Job drawing, mm, ordinate dimensions from the low corner. One solid piece. A direction names the side the tool comes from. Give positions to 0.01 mm unless a question says otherwise; leave off trailing zeros. Write each loop counter-clockwise with the first axis right and the second up, starting at its lowest first coordinate (ties: lowest second). Pieces come first, ordered by that corner, then holes. Notation, with made-up numbers: (18, 16.25) - (45, 16.25) arc R16 cw to (45, 39.25) - close; hole circle Ø8 at (-13.5, 37). An arc over 180 degrees is marked (long way). Answer in a Markdown table with one row per item. Add a question column.
1. Band-saw the part on C-C on z = 8. Write the cut outline in (x, y).
2. Pull direction Y, two halves, no side cores. Call the marked faces 1, 2 and 3: released by +Y, released by -Y, zero draft, split by the parting line, or undercut.
3. Band-saw the part on A-A on x = 15. Write the cut outline in (y, z), plus the area to 3 significant figures.
4. Which spindle directions (+Z, -Z, +X, -X, +Y, -Y) get a long thin tool onto all of the face, cutting with end or side? Do the marked faces 4 and 5. Say none if no direction does.
5. Band-saw the part on B-B on y = 29. Write the cut outline in (x, z).
6. Probe line 1 along X through (y, z) = (55.5, 4.75); line 2 along Y through (x, z) = (158, 13); line 3 along X through (y, z) = (86, 1.5). List the from-to ranges inside material, lowest first.
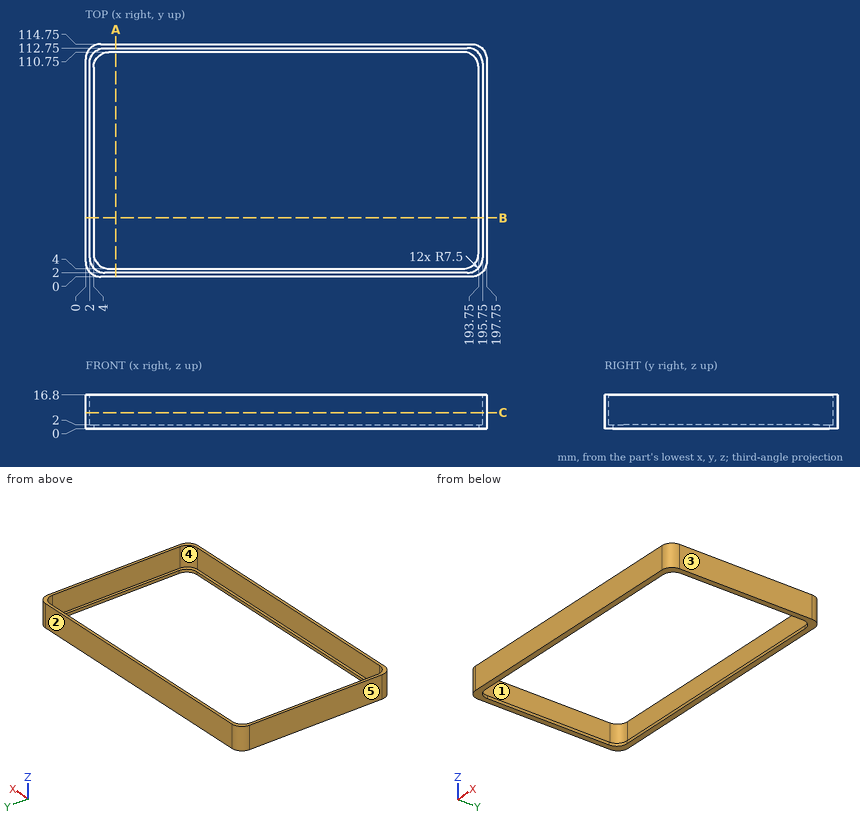
Values:
| question | item | result |
|---|---|---|
| 1 | outline | (0, 7.5) arc R7.5 ccw to (7.5, 0) - (190.25, 0) arc R7.5 ccw to (197.75, 7.5) - (197.75, 107.25) arc R7.5 ccw to (190.25, 114.75) - (7.5, 114.75) arc R7.5 ccw to (0, 107.25) - close; hole (2, 9.5) arc R7.5 ccw to (9.5, 2) - (188.25, 2) arc R7.5 ccw to (195.75, 9.5) - (195.75, 105.25) arc R7.5 ccw to (188.25, 112.75) - (9.5, 112.75) arc R7.5 ccw to (2, 105.25) - close |
| 2 | face 1 | undercut |
| 2 | face 2 | released by +Y |
| 2 | face 3 | zero draft |
| 3 | outline | (0, 0) - (4, 0) - (4, 2) - (2, 2) - (2, 16.8) - (0, 16.8) - close; (110.75, 0) - (114.75, 0) - (114.75, 16.8) - (112.75, 16.8) - (112.75, 2) - (110.75, 2) - close |
| 3 | area | 75.2 mm² |
| 4 | face 4 | +Z |
| 4 | face 5 | +Z, -Z, -X, +Y, -Y |
| 5 | outline | (0, 0) - (4, 0) - (4, 2) - (2, 2) - (2, 16.8) - (0, 16.8) - close; (193.75, 0) - (197.75, 0) - (197.75, 16.8) - (195.75, 16.8) - (195.75, 2) - (193.75, 2) - close |
| 6 | line 1 | x = 0 to 2, 195.75 to 197.75 |
| 6 | line 2 | y = 0 to 2, 112.75 to 114.75 |
| 6 | line 3 | x = 0 to 4, 193.75 to 197.75 |
